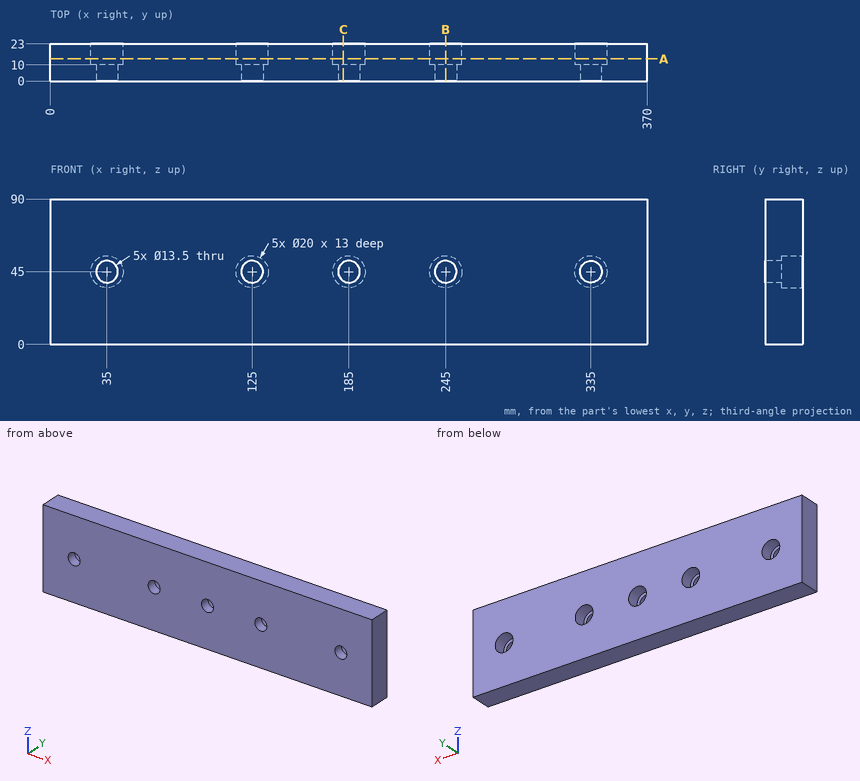
Answer from the drawing. Dimensions are ordinates in mm from the lowest x, y and z of the part. Round coordinates to 2 decimals unless told otherwise and drop trailing zeros. Order: outer loops, then holes, each group sorted by start corner. A loop starts at its lowest first (then second) coordinate and runs counter-clockwise, first axis right, second up. Notation, with made-up numbers: (60.5, -29.5) - (90.5, -29.5) arc R13 ccw to (90.5, -24.5) - close; hole circle Ø11 at (21.5, 44.25). An arc over 180 degrees is marked (long way). Put each result on its own line as item: value. Start each with the question number.
(1) Find section B-B (x = 245). Give the vertices of the cut face in (y, z).
(2) Find section A-A (y = 13.75). Give the vertices of the cut face in (x, z).
(3) Find section C-C (x = 181.5). Give the vertices of the cut face in (y, z).
(4) Straight lines are drawn through the part: probe 1 along X at (y, z) = (17.5, 45); probe 2 along X at (y, z) = (4.75, 45); probe 3 along Z at (x, y) = (245, 3). For each, find the intervals that lie inside material, in ascending order. Write a range as from..to.
(5) Given P1, Ø16, axis at x = 335, z = 45, coming from the +Y side, flat-ended and moving along its own axis, determine where the tip first touches the part or whether it passes through.
Reply:
1. outline: (0, 0) - (23, 0) - (23, 35) - (10, 35) - (10, 38.25) - (0, 38.25) - close; (0, 51.75) - (10, 51.75) - (10, 55) - (23, 55) - (23, 90) - (0, 90) - close
2. outline: (0, 0) - (370, 0) - (370, 90) - (0, 90) - close; hole circle Ø20 at (35, 45); hole circle Ø20 at (125, 45); hole circle Ø20 at (185, 45); hole circle Ø20 at (245, 45); hole circle Ø20 at (335, 45)
3. outline: (0, 0) - (23, 0) - (23, 35.63) - (10, 35.63) - (10, 39.23) - (0, 39.23) - close; (0, 50.77) - (10, 50.77) - (10, 54.37) - (23, 54.37) - (23, 90) - (0, 90) - close
4. probe 1: 0..25, 45..115, 135..175, 195..235, 255..325, 345..370
4. probe 2: 0..28.25, 41.75..118.25, 131.75..178.25, 191.75..238.25, 251.75..328.25, 341.75..370
4. probe 3: 0..38.25, 51.75..90
5. P1: y = 10
